Autodesk Fusion 360 part; units mm, degrees
sketch "Sketch1" plane through (0, 0, 0) normal (0, 1, 0) x (1, 0, 0)
  line L0 (0, -10) -> (54, -10)
  line L1 (54, -10) -> (54, -14)
  line L2 (54, -14) -> (0, -14)
  line L3 (0, -14) -> (0, -10)
  line L4 (0, -10) -> (1.5, -10)
  line L5 (1.5, -11) -> (1.5, -12.5)
  line L6 (1.5, -14) -> (0, -14)
  line L7 (0, -14) -> (0, -10)
  line L8 (54, -10) -> (52.5, -10)
  line L9 (52.5, -11) -> (52.5, -12.5)
  line L10 (52.5, -14) -> (54, -14)
  line L11 (54, -14) -> (54, -10)
  line L12 (1.5, -14) -> (52.5, -14)
  line L13 (52.5, -12.5) -> (1.5, -12.5)
  line L14 (1.5, -10) -> (4, -10)
  line L15 (4, -10) -> (4, -11)
  line L16 (4, -11) -> (1.5, -11)
  line L17 (52.5, -10) -> (50, -10)
  line L18 (50, -10) -> (50, -11)
  line L19 (50, -11) -> (52.5, -11)
  dimension "d1" = 54
  dimension "d2" = 4
  dimension "d3" = 1.5
  dimension "d4" = 1.5
  dimension "d5" = 51
  dimension "d6" = 1.5
extrude "Extrude1" add sketch "Sketch1" along normal blind 120 contours L0 L1 L2 L3 L4 L5 L6 L7 L8 L9 L10 L11 L12 L13 L14 L15 L16 L17 L18 L19
sketch "Sketch2" plane through (0, 0, 0) normal (0, -1, 0) x (1, 0, 0)
  line L0 (54, 14) -> (0, 14)
  line L1 (0, 14) -> (0, 10)
  line L2 (0, 10) -> (4, 10)
  line L3 (4, 10) -> (4, 11)
  line L4 (4, 11) -> (1.5, 11)
  line L5 (1.5, 11) -> (1.5, 12.5)
  line L6 (1.5, 12.5) -> (52.5, 12.5)
  line L7 (52.5, 12.5) -> (52.5, 11)
  line L8 (52.5, 11) -> (50, 11)
  line L9 (50, 11) -> (50, 10)
  line L10 (50, 10) -> (54, 10)
  line L11 (54, 10) -> (54, 14)
  line L12 (0, 0) -> (54, 0)
  line L13 (54, 0) -> (54, 25)
  line L14 (54, 25) -> (0, 25)
  line L15 (0, 25) -> (0, 0)
extrude "Extrude2" add sketch "Sketch2" along normal blind 2
sketch "Sketch3" plane through (0, 120, 0) normal (0, 1, 0) x (-1, 0, 0)
  line L0 (0, 14) -> (-54, 14)
  line L1 (-54, 14) -> (-54, 10)
  line L2 (-54, 10) -> (-50, 10)
  line L3 (-50, 10) -> (-50, 11)
  line L4 (-50, 11) -> (-52.5, 11)
  line L5 (-52.5, 11) -> (-52.5, 12.5)
  line L6 (-52.5, 12.5) -> (-1.5, 12.5)
  line L7 (-1.5, 12.5) -> (-1.5, 11)
  line L8 (-1.5, 11) -> (-4, 11)
  line L9 (-4, 11) -> (-4, 10)
  line L10 (-4, 10) -> (0, 10)
  line L11 (0, 10) -> (0, 14)
  line L12 (-1.5, 12.5) -> (-52.5, 12.5)
  line L13 (-52.5, 12.5) -> (-52.5, 13)
  line L14 (-52.5, 13) -> (-1.5, 13)
  line L15 (-1.5, 13) -> (-1.5, 12.5)
  dimension "d11" = 0.5
extrude "Extrude3" cut sketch "Sketch3" against normal blind 120 contours L6 L12 L13 L14 L15
sketch "Sketch4" plane through (0, 120, 0) normal (0, 1, 0) x (-1, 0, 0)
  line L0 (-1.5, 13) -> (-1.5, 11)
  line L1 (-1.5, 11) -> (-4, 11)
  line L2 (-4, 11) -> (-4, 10)
  line L3 (-4, 10) -> (0, 10)
  line L4 (0, 10) -> (0, 14)
  line L5 (0, 14) -> (-54, 14)
  line L6 (-54, 14) -> (-54, 10)
  line L7 (-54, 10) -> (-50, 10)
  line L8 (-50, 10) -> (-50, 11)
  line L9 (-50, 11) -> (-52.5, 11)
  line L10 (-52.5, 11) -> (-52.5, 13)
  line L11 (-52.5, 13) -> (-1.5, 13)
Geometry check sheet. Reference: the model listing, model coordinates, mm. A direction names the side the tool comes from. Give positions to 0.01 mm unless a question says otherwise; leave off trailing zeros. Loops run counter-clockwise (first coordinate to the right, second up) from the corner with the lowest first, then second, coordinate; pieces in that order, holes last.
(1) Section check C-C on z = 21.75. Record the cut outline in (x, y).
From the geometry:
outline: (0, -2) - (54, -2) - (54, 0) - (0, 0) - close
(2) Section check A-A on x = 19.5. Record the cut outline in (y, z), then the cut area to 3 significant figures.
From the geometry:
outline: (-2, 0) - (0, 0) - (0, 13) - (120, 13) - (120, 14) - (0, 14) - (0, 25) - (-2, 25) - close
area: 170 mm2
(3) Depth check by flat-ended pin: pin 1 Ø8 at (x, y) = (20, 13.5) entering from -Z; pin 2 Ø0.8 at (x, y) = (2.5, 60.5) entering from +Z; pin 3 Ø4.5 at (x, y) = (52, 34) entering from -Z. Enter the tip coordinate at first touch or a pass-through.
From the geometry:
pin 1: stops at z = 13
pin 2: stops at z = 14
pin 3: stops at z = 10
(4) Section check B-B on y = 17. Record the cut outline in (x, z).
From the geometry:
outline: (0, 10) - (4, 10) - (4, 11) - (1.5, 11) - (1.5, 13) - (52.5, 13) - (52.5, 11) - (50, 11) - (50, 10) - (54, 10) - (54, 14) - (0, 14) - close
(5) Set-up check for faces 4 (the flat face through (54, 59, 12)), 5 (the flat face through (27, 59, 14)), 6 (the flat face through (2, 59, 10)), 7 (the flat face through (51, 59, 11)): record each of +Z, -Z, +X, -X, +Y, -Y from which the full face is reachable in a straight line by a thin tool's end or side.
From the geometry:
face 4: +Z, -Z, +X, +Y, -Y
face 5: +Z, +X, -X, +Y
face 6: -Z, +X, -X, +Y
face 7: +Y
(6) Thickness scan on L1, parallel to Z at x = 51, y = 49.5; L2, parallel to Y at x = 35.5, z = 3; L3, parallel to Z at x = 36, y = 15. Record the ranges inside material, lowest first.
From the geometry:
L1: z = 10 to 11, 13 to 14
L2: y = -2 to 0
L3: z = 13 to 14
(7) Release check for a two-part mould opening along Z. For faces 1 (the flat face through (52, 59, 10)), 2 (the flat face through (3, 59, 11)), 3 (the flat face through (27, -2, 13)) record: released by +Z, released by -Z, zero draft, split by the parting line, or undercut.
From the geometry:
face 1: released by -Z
face 2: undercut
face 3: zero draft
